Geometry check sheet. Reference: drawing and pictorial views, mm from the part's lowest x, y, z. A direction names the side the tool comes from. Coordinates: 2 decimals unless noted, no trailing zeros. Loops run counter-clockwise (first coordinate to the right, second up) from the corner with the lowest first, then second, coordinate; pieces in that order, holes last. Notation, with made-up numbers: (89, 41) - (112, 41) arc R31 cw to (112, 73) - close; hole circle Ø1 at (73.25, -13). An arc over 180 degrees is marked (long way). One line per item, written item: value.
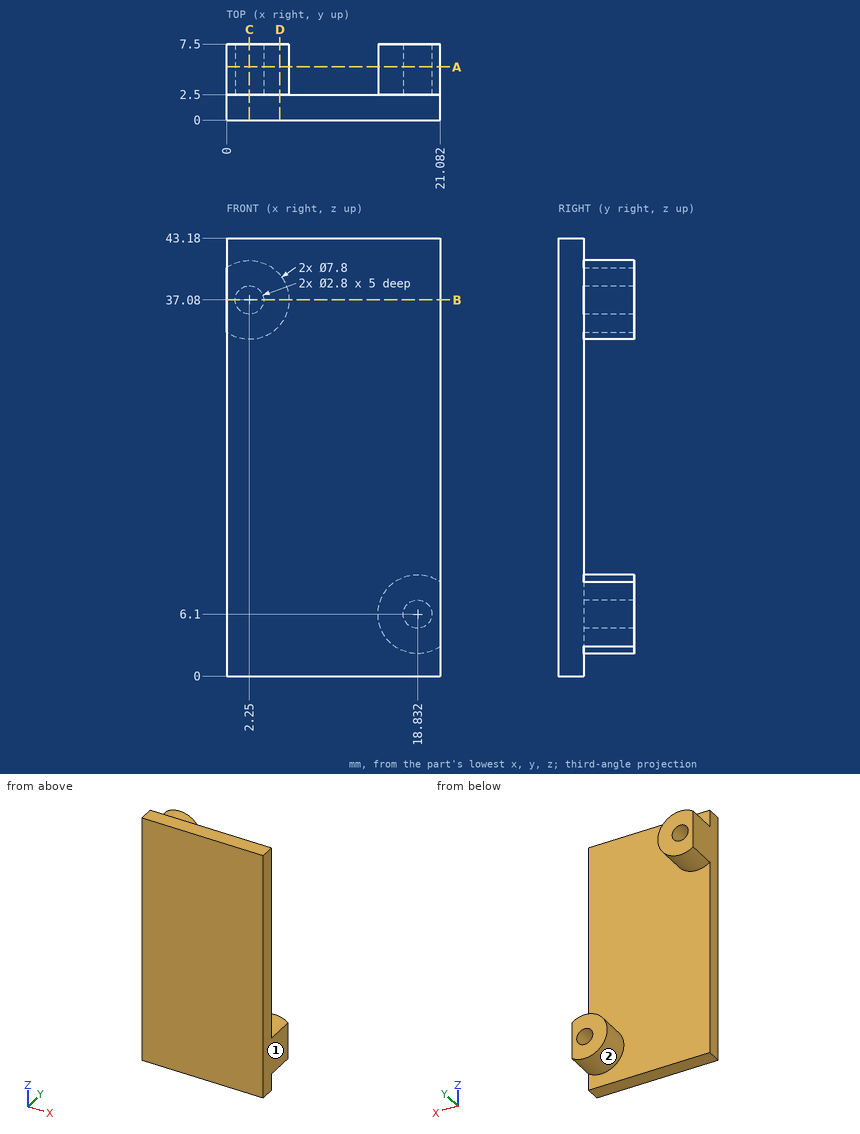
(1) Cross-section at C-C on x = 2.25. Record the cut outline in (y, z).
Reply:
outline: (0, 0) - (2.5, 0) - (2.5, 33.18) - (7.5, 33.18) - (7.5, 35.68) - (2.5, 35.68) - (2.5, 38.48) - (7.5, 38.48) - (7.5, 40.98) - (2.5, 40.98) - (2.5, 43.18) - (0, 43.18) - close
(2) Cross-section at B-B on z = 37.08. Record the cut outline in (x, y), and give its area (3 significant figures).
Reply:
outline: (0, 0) - (21.08, 0) - (21.08, 2.5) - (6.15, 2.5) - (6.15, 7.5) - (3.65, 7.5) - (3.65, 2.5) - (0.85, 2.5) - (0.85, 7.5) - (0, 7.5) - close
area: 69.5 mm2
(3) Cross-section at D-D on x = 5.25. Record the cut outline in (y, z).
Reply:
outline: (0, 0) - (2.5, 0) - (2.5, 34.59) - (7.5, 34.59) - (7.5, 39.57) - (2.5, 39.57) - (2.5, 43.18) - (0, 43.18) - close
(4) Go/stop test with a flat-tipped pin: pin 1 Ø2 at (x, z) = (18, 28) entering from +Y. Record where the tip stops, or that it passes through.
Reply:
pin 1: y = 2.5
(5) Access from +Z, -Z, +X, -X, +Y, -Y to the whole of each face (thin tool, end or side, straight path). Record for the marked faces 1 and 2.
Reply:
face 1: +Z, -Z, +X, +Y, -Y
face 2: +Y
(6) Cross-section at A-A on y = 5.25. Record the cut outline in (x, z).
Reply:
outline: (0, 33.89) arc R3.9 ccw (long way) to (0, 40.27) - close; (21.08, 2.91) - (21.08, 9.29) arc R3.9 ccw (long way) to start; hole circle Ø2.8 at (2.25, 37.08); hole circle Ø2.8 at (18.83, 6.1)
(7) Material ranges on probe 1 along X at (y, z) = (6.1, 37.08); probe 2 along Y at (x, z) = (18.5, 34); probe 3 along Z at (x, y) = (16.25, 5.25), recorded low to high. Write a range as from..to.
Reply:
probe 1: 0..0.85, 3.65..6.15
probe 2: 0..2.5
probe 3: 3.18..9.02
